Build history of the part. All positions in model axes, mm. Round coordinates to 2 decimals unless told otherwise and drop trailing zeros. Write each loop counter-clockwise with the first axis right and the second up, starting at its lowest first coordinate (ties: lowest second). Pieces come first, ordered by that corner, then holes. Notation, with made-up numbers: (24, 70.5) - (63, 70.5) arc R37 cw to (63, 108.5) - close; hole circle Ø3 at (-32, -10.75). An arc over 180 degrees is marked (long way). One line per question, with ' | ' between items.
from build123d import *

# Parameters (mm, degrees)
SKETCH_1_R      = 5
SKETCH_1_R_2    = 1.75
EXTRUDE_1_DEPTH = 3
CHAMFER_1_SIZE  = 1.75
FILLET_1_R      = 0.2


with BuildPart() as part:
    # Эскиз1 → Бобышка-Вытянуть1 (new body)
    with BuildSketch(Plane(origin=(0, 0, 0), x_dir=(1, 0, 0), z_dir=(0, 1, 0))):
        with Locations(Location((0, 0, 0), (0, 0, 270))):
            Circle(SKETCH_1_R)
        with Locations(Location((0, 0, 0), (0, 0, 270))):
            Circle(SKETCH_1_R_2, mode=Mode.SUBTRACT)
    extrude(amount=EXTRUDE_1_DEPTH)

    # Фаска1
    chamfer_1_edges = [part.edges().sort_by_distance(p)[0] for p in [
        (0, 3, -1.75),
    ]]
    chamfer(chamfer_1_edges, length=CHAMFER_1_SIZE)

    # Скругление1
    fillet_1_edges = [part.edges().sort_by_distance(p)[0] for p in [
        (0, 3, -3.5),
        (0, 0, -5),
        (0, 3, -5),
        (0, 1.25, -1.75),
    ]]
    fillet(fillet_1_edges, radius=FILLET_1_R)


solid = part.part
Q1. Drop flat-ended pins along their axis: pin 1 (5 mm diameter, centred on x = -2, z = -3.5, fed in from -Y); pin 2 (1 mm diameter, centred on x = 4, y = 0.5, fed in from +Z). Give the stop position or say it passes through.
Found:
pin 1: y = 0 | pin 2: z = 3.57
Q2. Saw through at A-A, the plane y = 2.35. List the corners of the cut face in (x, z).
Found:
outline: circle Ø10 at (0, 0); hole circle Ø5.7 at (0, 0)
Q3. Pull direction X, two halves, no side cores. Call faces 1 (the flat face through (0, 0, 2)), 2 (the cylindrical face through (-4.88, 1.48, -1.08)), 3 (the cylindrical face through (-1.71, 0.58, -0.38)): +X half, -X half, draft (parallel to the pull), parting line (faces both ways), or undercut.
Found:
face 1: draft | face 2: parting line | face 3: undercut
Q4. Saw through at B-B, the plane y = 1. List the corners of the cut face in (x, z).
Found:
outline: circle Ø10 at (0, 0); hole circle Ø3.5 at (0, 0)
Q5. Drill centre lines: L1, parallel to X at y = 0.95, z = 0; L2, parallel to Z at x = 2, y = 1.8; L3, parallel to X at y = 2.05, z = 1. Where is each one in solid material? Low to high. Write a range as from..to.
Found:
L1: -5..-1.75, 1.75..5 | L2: -4.58..-1.14, 1.14..4.58 | L3: -4.9..-2.35, 2.35..4.9
